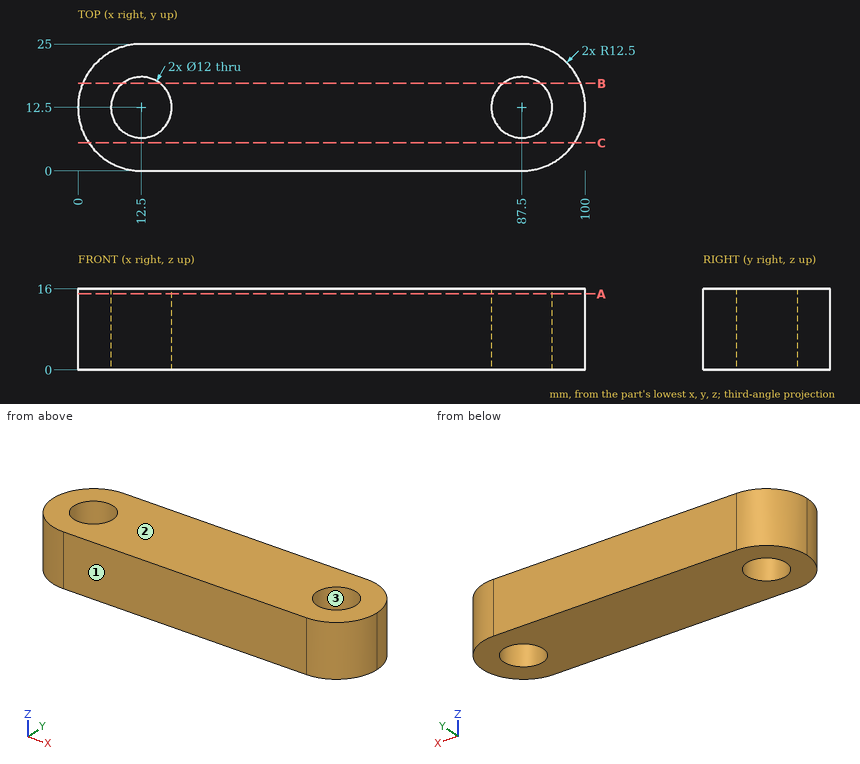
Can you work these out from the drawing? Everything is in mm from the part's minimum corner. Round coordinates to 2 decimals unless told otherwise and drop trailing zeros. Loops run counter-clockwise (first coordinate to the right, second up) from the corner with the lowest first, then second, coordinate; pieces in that order, holes last. Notation, with made-up numbers: (44, 35.5) - (64, 35.5) arc R26 cw to (64, 49.5) - close; hole circle Ø2 at (68, 54). An arc over 180 degrees is marked (long way). Write item = value, one per line. Start each with the question number.
(1) If we section it at B-B (y = 17.25): Please give me the cut outline in (x, z), and give its area (3 significant figures).
(2) If we mould it in two halves opening along Y, with no side actions, what happens to the marked faces 1, 2 and 3? For each: released by +Y, released by -Y, zero draft, split by the parting line, or undercut.
(3) For P1, Ø7, axis at x = 12.5, y = 12.5, coming from the -Z side; P2, Ø5, axis at y = 14, z = 13.5, coming from the -X side; P3, Ø3, axis at y = 17, z = 4, coming from the +X side, each with a flat end and sliding along its axis, tell me the tip position at first contact or that it passes through.
(4) If we section it at C-C (y = 5.5): Please give me the cut outline in (x, z).
(5) If we section it at A-A (z = 15): Please give me the cut outline in (x, y), and give its area (3 significant figures).
(6) If I drill on probe 1 along X at (y, z) = (13.25, 14.75); probe 2 along X at (y, z) = (10.5, 11.5); probe 3 along Y at (x, z) = (12.5, 4), over which ranges is the centre line in solid material (lowest first)? Write a range as [from, to].
Ans:
q1.outline = (0.94, 0) - (8.83, 0) - (8.83, 16) - (0.94, 16) - close; (16.17, 0) - (83.83, 0) - (83.83, 16) - (16.17, 16) - close; (91.17, 0) - (99.06, 0) - (99.06, 16) - (91.17, 16) - close
q1.area = 1,340 mm²
q2.face_1 = released by -Y
q2.face_2 = zero draft
q2.face_3 = undercut
q3.P1 = through
q3.P2 = 0
q3.P3 = 99.63
q4.outline = (2.14, 0) - (97.86, 0) - (97.86, 16) - (2.14, 16) - close
q5.outline = (12.5, 0) - (87.5, 0) arc R12.5 ccw to (87.5, 25) - (12.5, 25) arc R12.5 ccw to start; hole circle Ø12 at (12.5, 12.5); hole circle Ø12 at (87.5, 12.5)
q5.area = 2,140 mm²
q6.probe_1 = [0.02, 6.55], [18.45, 81.55], [93.45, 99.98]
q6.probe_2 = [0.16, 6.84], [18.16, 81.84], [93.16, 99.84]
q6.probe_3 = [0, 6.5], [18.5, 25]
